Part model, mm, in its own coordinate system. Face numbers are marked on the shaded views. Coordinates: 2 decimals unless noted, no trailing zeros. Order: outer loops, then holes, each group sorted by start corner. A loop starts at its lowest first (then second) coordinate and runs counter-clockwise, first axis right, second up. Notation, with made-up numbers: (48.5, 0) - (65.5, 0) arc R24 ccw to (65.5, 15) - close; hole circle Ø4 at (67, 44). An arc over 180 degrees is marked (long way). Use a Markdown table: item, result. Add a question column.
1) Saw through at C-C on z = -79. List the corners of the cut face in (x, y).
2) Two-plate mould, pull along Y, no slides. Class the marked faces 1, 2 and 3: +Y half, -Y half, draft (parallel to the pull), parting line (faces both ways), or undercut.
3) Drop a flat-ended pin along its axis: P1, Ø8, axis at x = 90.5, z = -10.5, coming from the +Y side. Give the stop position or say it passes through.
4) Saw through at D-D on z = -13. List the corners of the cut face in (x, y), then the cut area to 3 significant figures.
5) Saw through at A-A on y = 0. List the corners of the cut face in (x, z), then the cut area to 3 significant figures.
6) Wall check: L1, parallel to Y at x = 0, z = -52; L2, parallel to Y at x = 7, z = -43.5; L3, parallel to X at y = 4, z = -98.5. Give the ranges that are in metal, low to high. Write a range as [from, to].
7) Saw through at B-B on x = 0. List the corners of the cut face in (y, z).
```python
from build123d import *

# Parameters (mm, degrees)
F0_W     = 254
F0_H     = 254
F1_DEPTH = 103.632
F2_R     = 25.4
F4_D     = 50.8


with BuildPart() as f1:
    # F0 (on Top) → F1 (new body)
    with BuildSketch(Plane.XY):
        Rectangle(F0_W, F0_H)
    extrude(amount=-F1_DEPTH)

    # F2
    f2_edges = [f1.edges().sort_by_distance(p)[0] for p in [
        (-127, -127, -51.816),
        (0, 127, 0),
        (127, 127, -51.816),
        (127, -127, -51.816),
    ]]
    fillet(f2_edges, radius=F2_R)

    # F4 (through all)
    with Locations(Plane.XY):
        with Locations((0, 0)):
            Hole(F4_D / 2)


solid = f1.part
```
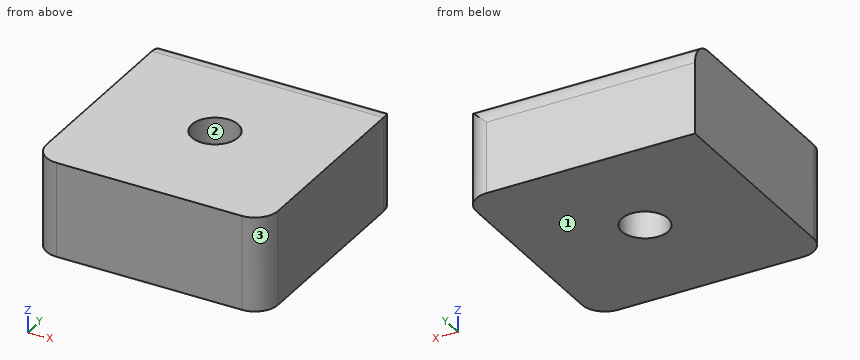
Results are:
| question | item | result |
|---|---|---|
| 1 | outline | (-127, -101.6) arc R25.4 ccw to (-101.6, -127) - (101.6, -127) arc R25.4 ccw to (127, -101.6) - (127, 101.6) arc R25.4 ccw to (101.6, 127) - (-127, 127) - close; hole circle Ø50.8 at (0, 0) |
| 2 | face 1 | draft |
| 2 | face 2 | undercut |
| 2 | face 3 | -Y half |
| 3 | P1 | y = 124.54 |
| 4 | outline | (-127, -101.6) arc R25.4 ccw to (-101.6, -127) - (101.6, -127) arc R25.4 ccw to (127, -101.6) - (127, 101.6) arc R25.4 ccw to (114, 123.77) - (-127, 123.77) - close; hole circle Ø50.8 at (0, 0) |
| 4 | area | 61,300 mm2 |
| 5 | outline | (-127, -103.63) - (-25.4, -103.63) - (-25.4, 0) - (-127, 0) - close; (25.4, -103.63) - (127, -103.63) - (127, 0) - (25.4, 0) - close |
| 5 | area | 21,100 mm2 |
| 6 | L1 | [-127, -25.4], [25.4, 127] |
| 6 | L2 | [-127, -24.42], [24.42, 127] |
| 6 | L3 | [-127, -25.08], [25.08, 127] |
| 7 | outline | (-127, -103.63) - (-25.4, -103.63) - (-25.4, 0) - (-127, 0) - close; (25.4, -103.63) - (127, -103.63) - (127, -25.4) arc R25.4 ccw to (101.6, 0) - (25.4, 0) - close |
